Geometry: final body of the model. Coordinates: model frame, mm. A direction names the side the tool comes from. Round coordinates to 2 decimals unless told otherwise and drop trailing zeros. Loops run counter-clockwise (first coordinate to the right, second up) from the corner with the lowest first, then second, coordinate; pieces in that order, holes last. Notation, with made-up numbers: M 49.25,81.25 L 90.25,81.25 A20 ccw 90.25,92.25 Z; hole C -13,23 d5. An arc over 180 degrees is marked long. Answer as a JSON object with one key per item and string values.
from build123d import *

# Parameters (mm, degrees)
F1_DEPTH = 3.048


with BuildPart() as f1:
    # F0 (on Front) → F1 (new body)
    with BuildSketch(Plane.XZ):
        with BuildLine():
            Line((7.9375, 0), (3.175, 0))
            ThreePointArc((3.175, 0), (-2.2450640303, -2.2450640303), (0, 3.175))
            Line((0, 3.175), (0, 7.9375))
            ThreePointArc((0, 7.9375), (-5.6126600757, 5.6126600757), (-7.9375, 0))
            ThreePointArc((-7.9375, 0), (-5.6126600757, -5.6126600757), (0, -7.9375))
            ThreePointArc((0, -7.9375), (5.6126600757, -5.6126600757), (7.9375, 0))
        make_face()
        with BuildLine():
            Line((8.9296875, 7.9375), (7.9375, 0))
            Line((7.9375, 0), (36.5125, 0))
            ThreePointArc((36.5125, 0), (38.8373399243, 5.6126600757), (44.45, 7.9375))
            Line((44.45, 7.9375), (9.9234625, 7.9375))
            Line((9.9234625, 7.9375), (8.9296875, 7.9375))
        make_face()
        with BuildLine():
            Line((36.5125, 0), (7.9375, 0))
            ThreePointArc((7.9375, 0), (5.6126600757, -5.6126600757), (0, -7.9375))
            Line((0, -7.9375), (44.45, -7.9375))
            ThreePointArc((44.45, -7.9375), (38.8373399243, -5.6126600757), (36.5125, 0))
        make_face()
        with BuildLine():
            ThreePointArc((0, 7.9375), (5.6126600757, 5.6126600757), (7.9375, 0))
            Line((7.9375, 0), (8.9296875, 7.9375))
            Line((8.9296875, 7.9375), (0, 7.9375))
        make_face()
        with BuildLine():
            ThreePointArc((-7.9375, 0), (-5.6126600757, 5.6126600757), (0, 7.9375))
            Line((0, 7.9375), (0, 47.625))
            ThreePointArc((0, 47.625), (-9.7463072395, 50.9690335492), (-15.3865384615, 59.5923076923))
            Line((-15.3865384615, 59.5923076923), (-7.9375, 0))
        make_face()
        with BuildLine():
            Line((0, 47.625), (0, 7.9375))
            Line((0, 7.9375), (8.9296875, 7.9375))
            Line((8.9296875, 7.9375), (15.3865384615, 59.5923076923))
            ThreePointArc((15.3865384615, 59.5923076923), (9.7463072395, 50.9690335492), (0, 47.625))
        make_face()
        with BuildLine():
            ThreePointArc((44.45, 7.9375), (38.8373399243, 5.6126600757), (36.5125, 0))
            ThreePointArc((36.5125, 0), (38.8373399243, -5.6126600757), (44.45, -7.9375))
            ThreePointArc((44.45, -7.9375), (50.0626600757, -5.6126600757), (52.3875, 0))
            ThreePointArc((52.3875, 0), (50.0626600757, 5.6126600757), (44.45, 7.9375))
        make_face()
        with BuildLine():
            ThreePointArc((47.625, 0), (44.45, -3.175), (41.275, 0))
            ThreePointArc((41.275, 0), (44.45, 3.175), (47.625, 0))
        make_face(mode=Mode.SUBTRACT)
        with BuildLine():
            ThreePointArc((-15.3865384615, 59.5923076923), (-9.7463072395, 50.9690335492), (0, 47.625))
            Line((0, 47.625), (0, 60.325))
            ThreePointArc((0, 60.325), (-3.175, 63.5), (0, 66.675))
            Line((0, 66.675), (0, 79.375))
            ThreePointArc((0, 79.375), (-10.4912828548, 75.4142187767), (-15.7474569047, 65.5082893304))
            ThreePointArc((-15.7474569047, 65.5082893304), (-15.8430821396, 64.5061676396), (-15.875, 63.5))
            Line((-15.875, 63.5), (-15.3865384615, 59.5923076923))
        make_face()
        with BuildLine():
            Line((0, 60.325), (0, 47.625))
            ThreePointArc((0, 47.625), (9.7463072395, 50.9690335492), (15.3865384615, 59.5923076923))
            Line((15.3865384615, 59.5923076923), (15.875, 63.5))
            Line((15.875, 63.5), (15.3865384615, 67.4076923077))
            ThreePointArc((15.3865384615, 67.4076923077), (9.7463072395, 76.0309664508), (0, 79.375))
            Line((0, 79.375), (0, 66.675))
            ThreePointArc((0, 66.675), (2.2450640303, 65.7450640303), (3.175, 63.5))
            ThreePointArc((3.175, 63.5), (2.2450640303, 61.2549359697), (0, 60.325))
        make_face()
        with BuildLine():
            Line((15.875, 63.5), (15.3865384615, 59.5923076923))
            ThreePointArc((15.3865384615, 59.5923076923), (15.7524112928, 61.5309485884), (15.875, 63.5))
        make_face()
        with BuildLine():
            ThreePointArc((-15.875, 63.5), (-15.7524112928, 61.5309485884), (-15.3865384615, 59.5923076923))
            Line((-15.3865384615, 59.5923076923), (-15.875, 63.5))
        make_face()
        with BuildLine():
            Line((15.3865384615, 67.4076923077), (15.875, 63.5))
            ThreePointArc((15.875, 63.5), (15.7524112928, 65.4690514116), (15.3865384615, 67.4076923077))
        make_face()
        with BuildLine():
            ThreePointArc((0, 79.375), (9.7463072395, 76.0309664508), (15.3865384615, 67.4076923077))
            Line((15.3865384615, 67.4076923077), (9.525, 114.3))
            ThreePointArc((9.525, 114.3), (6.7351920908, 107.5648079092), (0, 104.775))
            Line((0, 104.775), (0, 79.375))
        make_face()
        with BuildLine():
            ThreePointArc((-15.7474569047, 65.5082893304), (-10.4912828548, 75.4142187767), (0, 79.375))
            Line((0, 79.375), (0, 104.775))
            ThreePointArc((0, 104.775), (-6.7351920908, 107.5648079092), (-9.525, 114.3))
            Line((-9.525, 114.3), (-15.7474569047, 65.5082893304))
        make_face()
        with BuildLine():
            ThreePointArc((0, 104.775), (6.7351920908, 107.5648079092), (9.525, 114.3))
            ThreePointArc((9.525, 114.3), (0, 123.825), (-9.525, 114.3))
            ThreePointArc((-9.525, 114.3), (-6.7351920908, 107.5648079092), (0, 104.775))
        make_face()
        with BuildLine():
            ThreePointArc((3.175, 114.3), (2.2450640303, 112.0549359697), (0, 111.125))
            ThreePointArc((0, 111.125), (-2.2450640303, 116.5450640303), (3.175, 114.3))
        make_face(mode=Mode.SUBTRACT)
    extrude(amount=F1_DEPTH)


solid = f1.part
1) Pin query (flat end, axial travel): P1, Ø1.5, axis at x = 4.5, y = -1, coming from the +Z side; P2, Ø1.5, axis at x = 28.5, y = -2, coming from the +Z side; P3, Ø1, axis at y = -2.5, z = 71.5, coming from the +X side; P4, Ø5.5, axis at x = 0, z = 114.3, coming from the +Y side. Return the tip coordinate at first contact, or that it passes through.
Results:
{"P1": "z = 123.06", "P2": "z = 7.94", "P3": "x = 14.94", "P4": "through"}
2) Section query C-C (z = 6). Return the cut outline in (x, y).
Results:
{"outline": "M -8.69,-3.05 L 0,-3.05 L 0,0 L -8.69,0 Z; M 5.2,-3.05 L 49.65,-3.05 L 49.65,0 L 5.2,0 Z"}
3) Ray query, line 1 (Z direction, x = -2, y = -2.65); line 2 (X direction, y = -1.7, z = 114.3) (3 decimals); line 3 (Z direction, x = 27, y = -2.1). Return the intervals inside material, ascending.
Results:
{"line 1": "-7.68 to -2.47, 2.47 to 61.03, 65.97 to 111.83, 116.77 to 123.61", "line 2": "-9.525 to -3.175, 3.175 to 9.525", "line 3": "-7.94 to 7.94"}
4) Pull-direction query (X, two-part tool) for faces 1 (the cylindrical face through (0.209, -1.503, 123.823)), 2 (the flat face through (3, -3.048, 59)), 3 (the flat face through (12.5, -1.5, 90.5)), 4 (the cylindrical face through (41.52, -1.5, -1.22)); classes: +X half, -X half, draft (parallel to the pull), parting line (faces both ways), or undercut.
Results:
{"face 1": "parting line", "face 2": "draft", "face 3": "+X half", "face 4": "undercut"}
5) Section query D-D (z = 51). Return the cut outline in (x, y).
Results:
{"outline": "M -14.31,-3.05 L 14.31,-3.05 L 14.31,0 L -14.31,0 Z"}
6) Section query A-A (y = -0.6). Count the separate pieces of the cut face and the enclosed holes in it, and give its area (3 significant figures).
Results:
{"separate pieces": "1", "enclosed holes": "4", "area": "3,570 mm2"}
7) Section query B-B (x = 6). Return the cut outline in (y, z).
Results:
{"outline": "M -3.05,-7.94 L 0,-7.94 L 0,0 L -3.05,0 Z; M -3.05,5.2 L 0,5.2 L 0,121.7 L -3.05,121.7 Z"}
8) Reachability of faces 5 (the cylindrical face through (-5.674, -1.503, -5.551)), 6 (the flat face through (0, -2, 6)), 7 (the flat face through (27, -2, 7.938)) from +Z, -Z, +X, -X, +Y, -Y: full face, straight path, thin tool, end or side. Return the list, or none.
Results:
{"face 5": "-Z, -X, +Y, -Y", "face 6": "+Y, -Y", "face 7": "+X, +Y, -Y"}
